```python
from build123d import *


with BuildPart() as part:
    # Sketch1 → Revolve1 (revolve)
    with BuildSketch(Plane.XY, mode=Mode.PRIVATE) as revolve1_sk:
        with BuildLine():
            Line((15, 120), (0, 120))
            Line((0, 120), (0, 107.5))
            Line((0, 107.5), (5, 107.5))
            Line((5, 107.5), (9, 105))
            Line((9, 105), (12.8333335, 108.194444583))
            Line((12.8333335, 108.194444583), (12.8333335, 110))
            Line((12.8333335, 110), (10.666667, 110))
            ThreePointArc((10.666667, 110), (9, 108.333333), (7.333333, 110))
            Line((7.333333, 110), (5, 110))
            Line((5, 110), (5, 115))
            Line((5, 115), (15, 115))
            Line((15, 115), (15, 120))
        make_face()
    revolve(revolve1_sk.sketch.rotate(Axis((-0.005, 0, 0), (1, 0, 0)), 270), axis=Axis((-0.005, 0, 0), (1, 0, 0)))


solid = part.part
```
Input: part model. Units: mm. Frame: model coordinates. A direction names the side the tool comes from. Coordinates: 2 decimals unless noted, no trailing zeros. Loops run counter-clockwise (first coordinate to the right, second up) from the corner with the lowest first, then second, coordinate; pieces in that order, holes last. Notation, with made-up numbers: M 77.25,27.5 L 90.25,27.5 A18 ccw 90.25,47.5 Z; hole C -30,54.25 d1. An arc over 180 degrees is marked long. Use a Markdown table: item, result. Add a question column.
1) Section A-A, the plane z = 0. Return the cut outline in (x, y), plus the area to 3 significant figures.
2) Pin query (flat end, axial travel): P1, Ø8, axis at x = 2, y = -64.5, coming from the -Z side; P2, Ø1, axis at x = 8, y = -54, coming from the -Z side; P3, Ø4, axis at x = 5, z = -58, coming from the -Y side. Return the tip coordinate at first contact, or that it passes through.
3) Set-up query: faces 5 (the cylindrical face through (2.535, -104.944, 23.304)), 6 (the cylindrical face through (11.73, -97.59, -50.76)), 7 (the flat face through (0, 45, 98)). Return all of +Z, -Z, +X, -X, +Y, -Y with unobstructed straight access to the full face (end or side cutting, diameter ignored); none if empty.
4) Draft query along Y for faces 1 (the cylindrical face through (10.07, -112.265, 24.93)), 2 (the cylindrical face through (6.15, -97.59, -50.76)), 3 (the cylindrical face through (7.395, 5.276, 119.884)), 4 (the flat face through (15, -8, 115)). Return one class per face: +Y half, -Y half, draft (parallel to the pull), parting line (faces both ways), or undercut.
5) Section C-C, the plane x = 2.75. Return the cut outline in (y, z), plus the area to 3 significant figures.
6) Line query: L1, parallel to Y at x = 6.5, z = -49; L2, parallel to Y at x = 2.7, z = 0; L3, parallel to Y at x = 8.75, z = 32.5. Output: solid intervals per line, ascending. Write a range as from..to.
Answer below:
| question | item | result |
|---|---|---|
| 1 | outline | M 0,-120 L 15,-120 L 15,-115 L 5,-115 L 5,-110 L 7.33,-110 A1.67 cw 10.67,-110 L 12.83,-110 L 12.83,-108.19 L 9,-105 L 5,-107.5 L 0,-107.5 Z; M 0,107.5 L 5,107.5 L 9,105 L 12.83,108.19 L 12.83,110 L 10.67,110 A1.67 cw 7.33,110 L 5,110 L 5,115 L 15,115 L 15,120 L 0,120 Z |
| 1 | area | 272 mm2 |
| 2 | P1 | z = -103.63 |
| 2 | P2 | z = -107.41 |
| 2 | P3 | y = -106.13 |
| 3 | face 5 | -X |
| 3 | face 6 | +X |
| 3 | face 7 | +Z, -Z, -X, +Y, -Y |
| 4 | face 1 | undercut |
| 4 | face 2 | undercut |
| 4 | face 3 | parting line |
| 4 | face 4 | draft |
| 5 | outline | C 0,0 d240; hole C 0,0 d215 |
| 5 | area | 8,930 mm2 |
| 6 | L1 | -109.54..-104.04, -98.48..-94.63, 94.63..98.48, 104.04..109.54 |
| 6 | L2 | -120..-107.5, 107.5..120 |
| 6 | L3 | -115.52..-110.31, -103.36..-100.01, 100.01..103.36, 110.31..115.52 |
